from build123d import *

# Parameters (mm, degrees)
F0_W     = 95.25
F0_H     = 76.2
F0_R     = 23.749
F1_DEPTH = 25.4
F3_D     = 7.3152


with BuildPart() as f1:
    # F0 (on Front) → F1 (new body)
    with BuildSketch(Plane.XZ):
        with Locations((14.847173, 7.273737)):
            Rectangle(F0_W, F0_H)
        with Locations((14.720173, 7.273737)):
            Circle(F0_R, mode=Mode.SUBTRACT)
    extrude(amount=F1_DEPTH)

    # F3 (through all)
    with Locations(Plane.XY.offset(45.373737)):
        with Locations((-24.527139, -12.7), (54.843643, -12.7)):
            Hole(F3_D / 2)


solid = f1.part
Geometry check sheet. Reference: the model listing, model coordinates, mm. Give positions to 0.01 mm unless a question says otherwise; leave off trailing zeros. Order: outer loops, then holes, each group sorted by start corner. A loop starts at its lowest first (then second) coordinate and runs counter-clockwise, first axis right, second up.
1. Sectioned sample at D-D (x = -7). Record the boundary of the cut face in (y, z).
Completed:
outline: (-25.4, -30.83) - (0, -30.83) - (0, -2.33) - (-25.4, -2.33) - close; (-25.4, 16.88) - (0, 16.88) - (0, 45.37) - (-25.4, 45.37) - close
2. Sectioned sample at B-B (x = 54). Record the boundary of the cut face in (y, z).
Completed:
outline: (-25.4, -30.83) - (-16.26, -30.83) - (-16.26, 45.37) - (-25.4, 45.37) - close; (-9.14, -30.83) - (0, -30.83) - (0, 45.37) - (-9.14, 45.37) - close
3. Sectioned sample at A-A (y = -14.5). Record the boundary of the cut face in (x, z), then the cut area to 3 significant figures.
Completed:
outline: (-32.78, -30.83) - (-27.71, -30.83) - (-27.71, 45.37) - (-32.78, 45.37) - close; (-21.34, -30.83) - (51.66, -30.83) - (51.66, 45.37) - (-21.34, 45.37) - close; (58.03, -30.83) - (62.47, -30.83) - (62.47, 45.37) - (58.03, 45.37) - close; hole circle Ø47.5 at (14.72, 7.27)
area: 4,520 mm2
4. Sectioned sample at C-C (y = -5.5). Record the boundary of the cut face in (x, z).
Completed:
outline: (-32.78, -30.83) - (62.47, -30.83) - (62.47, 45.37) - (-32.78, 45.37) - close; hole circle Ø47.5 at (14.72, 7.27)
5. Scan lines: line 1 (X direction, y = -10.75, z = -6.5); line 2 (X direction, y = -10.75, z = 31.5); line 3 (Z direction, x = 32.5, y = -6). Record each from-to range of solid material in increasing order.
Completed:
line 1: x = -32.78 to -27.62, -21.43 to -4.63, 34.07 to 51.75, 57.94 to 62.47
line 2: x = -32.78 to -27.62, -21.43 to 51.75, 57.94 to 62.47
line 3: z = -30.83 to -8.47, 23.02 to 45.37
6. Draft check along X on faces 1 (the face through (37.37, -12.52, 14.41)), 2 (the face through (14, -13, -30.826)), 3 (the face through (-27.906, -14.101, 6.74)), 4 (the face through (62.472, -13, 7)). Enter one of: pulls with the +X half, pulls with the -X half, needs draft (parallel to the pull), parting line crosses it, or undercut.
Completed:
face 1: undercut
face 2: needs draft
face 3: undercut
face 4: pulls with the +X half
